CAD build for the part. Positions are in the model's coordinates, mm. Round coordinates to 2 decimals unless told otherwise and drop trailing zeros. Order: outer loops, then holes, each group sorted by start corner. A loop starts at its lowest first (then second) coordinate and runs counter-clockwise, first axis right, second up. Notation, with made-up numbers: (36, 21.25) - (74, 21.25) arc R15 cw to (74, 44.25) - close; hole circle Ø7 at (-23.5, 53). An arc over 180 degrees is marked (long way). Use one line per item in the form item = value. Start each with the question number.
from build123d import *

# Parameters (mm, degrees)
BOSS_EXTRUDE1_DEPTH     = 25
CUT_EXTRUDE1_DEPTH      = 38.279220614
CIRPATTERN1_COUNT       = 8
SHELL2_T                = -10
BOSS_EXTRUDE2_DEPTH     = 15
SKETCH8_R               = 1.75
CUT_EXTRUDE3_DEPTH      = 3.89
SKETCH10_R              = 1.5
CUT_EXTRUDE5_DEPTH      = 10
CIRPATTERN2_COUNT       = 8
CUT_EXTRUDE7_DEPTH      = 2
CUT_EXTRUDE8_DEPTH      = 3.7
FILLET1_R               = 1
CUT_EXTRUDE9_DEPTH      = 1
SKETCH15_R              = 1.1
CUT_EXTRUDE11_DEPTH     = 4
MIRROR2_COPY_1_SKETCH_R = 1.1
MIRROR2_COPY_1_DEPTH    = 4
CUT_EXTRUDE12_DEPTH     = 2.5
SKETCH17_R              = 1
CUT_EXTRUDE13_DEPTH     = 4
CUT_EXTRUDE14_DEPTH     = 0.5
SKETCH19_R              = 3.8
CUT_EXTRUDE15_DEPTH     = 3
CIRPATTERN3_COUNT       = 8


with BuildPart() as part:
    # Sketch3 → Boss-Extrude1 (new body)
    with BuildSketch(Plane(origin=(0, 0, 0), x_dir=(1, 0, 0), z_dir=(0, 1, 0))):
        Polygon((-90, 37.279220614), (-90, -37.279220614), (0, 0), align=None)
    boss_extrude1 = extrude(amount=BOSS_EXTRUDE1_DEPTH)

    # Sketch4 → Cut-Extrude1 (cut, symmetric)
    with BuildSketch(Plane.XY):
        Polygon((-90, 25), (-90, 0), (-80, 25), align=None)
    cut_extrude1 = extrude(amount=CUT_EXTRUDE1_DEPTH, both=True, mode=Mode.SUBTRACT)

    # CirPattern1: Boss-Extrude1, Cut-Extrude1 ×8 about axis
    cirpattern1_axis = Axis((0, 0, 0), (0, 1, 0))
    for i in range(1, CIRPATTERN1_COUNT):
        add(boss_extrude1.rotate(cirpattern1_axis, i * 360 / CIRPATTERN1_COUNT))
        add(cut_extrude1.rotate(cirpattern1_axis, i * 360 / CIRPATTERN1_COUNT), mode=Mode.SUBTRACT)

    # Shell2
    shell2_openings = [part.faces().sort_by_distance(p)[0] for p in [
        (0, 0, 0),
    ]]
    offset(amount=SHELL2_T, openings=shell2_openings, kind=Kind.INTERSECTION)

    # Sketch5 → Boss-Extrude2 (add)
    with BuildSketch(Plane.XZ.offset(-15)):
        with BuildLine():
            Line((-79.229670386, -32.818004016), (-79.229670386, -26.828993349))
            ThreePointArc((-79.229670386, -26.828993349), (-70.654057407, -29.265868815), (-74.99480033, -37.052874072))
            Line((-74.99480033, -37.052874072), (-79.229670386, -32.818004016))
        make_face()
    boss_extrude2 = extrude(amount=BOSS_EXTRUDE2_DEPTH)

    # Sketch8 → Cut-Extrude3 (cut)
    with BuildSketch(Plane.XZ):
        with Locations((-75.906312549, -31.441424128)):
            Circle(SKETCH8_R)
    cut_extrude3 = extrude(amount=-CUT_EXTRUDE3_DEPTH, mode=Mode.SUBTRACT)

    # Sketch10 → Cut-Extrude5 (cut)
    with BuildSketch(Plane.XZ.offset(-3.89)):
        with Locations((-75.906312549, -31.441424128)):
            Circle(SKETCH10_R)
    cut_extrude5 = extrude(amount=-CUT_EXTRUDE5_DEPTH, mode=Mode.SUBTRACT)

    # CirPattern2: Boss-Extrude2, Cut-Extrude3, Cut-Extrude5 ×8 about axis
    cirpattern2_axis = Axis((0, 0, 0), (0, 1, 0))
    for i in range(1, CIRPATTERN2_COUNT):
        add(boss_extrude2.rotate(cirpattern2_axis, i * 360 / CIRPATTERN2_COUNT))
        add(cut_extrude3.rotate(cirpattern2_axis, i * 360 / CIRPATTERN2_COUNT), mode=Mode.SUBTRACT)
        add(cut_extrude5.rotate(cirpattern2_axis, i * 360 / CIRPATTERN2_COUNT), mode=Mode.SUBTRACT)

    # Sketch11 → Cut-Extrude7 (cut)
    with BuildSketch(Plane.XZ.offset(-15)):
        with BuildLine():
            Line((-34.358681844, -65.650070064), (34.041318156, -65.650070064))
            ThreePointArc((34.041318156, -65.650070064), (39.203197659, -63.511949566), (41.341318156, -58.350070064))
            Line((41.341318156, -58.350070064), (41.341318156, -19.050070064))
            ThreePointArc((41.341318156, -19.050070064), (39.203197659, -13.888190561), (34.041318156, -11.750070064))
            Line((34.041318156, -11.750070064), (-34.358681844, -11.750070064))
            ThreePointArc((-34.358681844, -11.750070064), (-39.520561346, -13.888190561), (-41.658681844, -19.050070064))
            Line((-41.658681844, -19.050070064), (-41.658681844, -58.350070064))
            ThreePointArc((-41.658681844, -58.350070064), (-39.520561346, -63.511949566), (-34.358681844, -65.650070064))
        make_face()
        Polygon((26.669250561, 70.01701088), (14.499741046, 57.72095305), (40.157988887, 32.326774235), (52.327498403, 44.622832065), align=None)
        Polygon((-45.807628052, 29.456027416), (-45.557628052, 30.956027416), (-50.265904305, 30.956027416), (-50.015904305, 29.456027416), (-61.961766178, 29.456027416), (-61.961766178, 13.460165542), (-63.461766178, 13.710165542), (-63.461766178, 9.001889289), (-61.961766178, 9.251889289), (-61.961766178, -6.743972584), (20.938233822, -6.743972584), (20.938233822, 10.356027416), (20.938233822, 10.513250754), (20.938233822, 12.198804078), (20.938233822, 12.356027416), (20.938233822, 29.456027416), (8.992371948, 29.456027416), (9.242371948, 30.956027416), (4.534095695, 30.956027416), (4.784095695, 29.456027416), align=None)
        with BuildLine():
            Line((45.394921968, -29.715967357), (66.654814344, -29.648319841))
            ThreePointArc((66.654814344, -29.648319841), (68.279008196, -28.969493954), (68.947484296, -27.341013079))
            Line((68.947484296, -27.341013079), (68.763251409, 30.558693813))
            ThreePointArc((68.763251409, 30.558693813), (68.084425523, 32.182887666), (66.455944648, 32.851363765))
            Line((66.455944648, 32.851363765), (45.196052273, 32.783716249))
            ThreePointArc((45.196052273, 32.783716249), (43.57185842, 32.104890363), (42.903382321, 30.476409488))
            Line((42.903382321, 30.476409488), (43.087615207, -27.423297405))
            ThreePointArc((43.087615207, -27.423297405), (43.766441094, -29.047491257), (45.394921968, -29.715967357))
        make_face()
        Polygon((8.912517718, 34.761532869), (9.383564949, 60.756265326), (-36.708868078, 61.591500425), (-37.179915309, 35.596767968), align=None)
    extrude(amount=-CUT_EXTRUDE7_DEPTH, mode=Mode.SUBTRACT)

    # Sketch13 → Cut-Extrude8 (cut)
    with BuildSketch(Plane.XZ.offset(-17)):
        with BuildLine():
            Line((34.041318156, -11.750070064), (-34.358681844, -11.750070064))
            ThreePointArc((-34.358681844, -11.750070064), (-39.520561346, -13.888190561), (-41.658681844, -19.050070064))
            Line((-41.658681844, -19.050070064), (-41.658681844, -58.350070064))
            ThreePointArc((-41.658681844, -58.350070064), (-39.520561346, -63.511949566), (-34.358681844, -65.650070064))
            Line((-34.358681844, -65.650070064), (34.041318156, -65.650070064))
            ThreePointArc((34.041318156, -65.650070064), (39.203197659, -63.511949566), (41.341318156, -58.350070064))
            Line((41.341318156, -58.350070064), (41.341318156, -19.050070064))
            ThreePointArc((41.341318156, -19.050070064), (39.203197659, -13.888190561), (34.041318156, -11.750070064))
        make_face()
    extrude(amount=-CUT_EXTRUDE8_DEPTH, mode=Mode.SUBTRACT)

    # Fillet1
    fillet1_edges = [part.edges().sort_by_distance(p)[0] for p in [
        (8.912517718, 16, 34.761532869),
        (-37.179915309, 16, 35.596767968),
        (-36.708868078, 16, 61.591500425),
        (9.383564949, 16, 60.756265326),
    ]]
    fillet(fillet1_edges, radius=FILLET1_R)

    # Sketch14 → Cut-Extrude9 (cut)
    with BuildSketch(Plane.XZ.offset(-17)):
        with BuildLine():
            Line((45.394921968, -29.715967357), (66.654814344, -29.648319841))
            ThreePointArc((66.654814344, -29.648319841), (68.279008196, -28.969493954), (68.947484296, -27.341013079))
            Line((68.947484296, -27.341013079), (68.763251409, 30.558693813))
            ThreePointArc((68.763251409, 30.558693813), (68.084425523, 32.182887666), (66.455944648, 32.851363765))
            Line((66.455944648, 32.851363765), (45.196052273, 32.783716249))
            ThreePointArc((45.196052273, 32.783716249), (43.57185842, 32.104890363), (42.903382321, 30.476409488))
            Line((42.903382321, 30.476409488), (43.087615207, -27.423297405))
            ThreePointArc((43.087615207, -27.423297405), (43.766441094, -29.047491257), (45.394921968, -29.715967357))
        make_face()
        Polygon((52.327498403, 44.622832065), (26.669250561, 70.01701088), (14.499741046, 57.72095305), (40.157988887, 32.326774235), align=None)
    extrude(amount=-CUT_EXTRUDE9_DEPTH, mode=Mode.SUBTRACT)

    # Sketch15 → Cut-Extrude11 (cut)
    with BuildSketch(Plane.XZ.offset(-18)):
        with Locations((65.616131079, 29.648675337)):
            Circle(SKETCH15_R)
    cut_extrude11 = extrude(amount=-CUT_EXTRUDE11_DEPTH, mode=Mode.SUBTRACT)

    # Mirror1: Cut-Extrude11 across plane
    add(cut_extrude11.mirror(Plane(origin=(-0.004422036, 0, 1.38973325), x_dir=(0.999994938, 0, 0.003181915), z_dir=(0.003181915, 0, -0.999994938))), mode=Mode.SUBTRACT)

    # Mirror2: Cut-Extrude11 across plane
    add(cut_extrude11.mirror(Plane(origin=(55.929855344, 0, 0.177964954), x_dir=(-0.003181915, 0, 0.999994938), z_dir=(-0.999994938, 0, -0.003181915))), mode=Mode.SUBTRACT)

    # Mirror2 copy 1 sketch → Mirror2 copy 1 (cut)
    with BuildSketch(Plane(origin=(111.850866616, 18, 3.135396408), x_dir=(-1, 0, 0), z_dir=(0, -1, 0))):
        with Locations((65.616131079, 29.648675337)):
            Circle(MIRROR2_COPY_1_SKETCH_R)
    extrude(amount=-MIRROR2_COPY_1_DEPTH, mode=Mode.SUBTRACT)

    # Sketch16 → Cut-Extrude12 (cut)
    with BuildSketch(Plane.XZ.offset(-17)):
        Polygon((4.784095695, 29.456027416), (-45.807628052, 29.456027416), (-45.557628052, 30.956027416), (-50.265904305, 30.956027416), (-50.015904305, 29.456027416), (-61.961766178, 29.456027416), (-61.961766178, 13.460165542), (-63.461766178, 13.710165542), (-63.461766178, 9.001889289), (-61.961766178, 9.251889289), (-61.961766178, -6.743972584), (20.938233822, -6.743972584), (20.938233822, 29.456027416), (8.992371948, 29.456027416), (9.242371948, 30.956027416), (4.534095695, 30.956027416), align=None)
    extrude(amount=-CUT_EXTRUDE12_DEPTH, mode=Mode.SUBTRACT)

    # Sketch17 → Cut-Extrude13 (cut)
    with BuildSketch(Plane.XZ.offset(-18)):
        with Locations((18.389142064, 57.67035938)):
            Circle(SKETCH17_R)
        with Locations((40.067163093, 36.21544376)):
            Circle(SKETCH17_R)
    extrude(amount=-CUT_EXTRUDE13_DEPTH, mode=Mode.SUBTRACT)

    # Sketch18 → Cut-Extrude14 (cut)
    with BuildSketch(Plane.XZ.offset(-17)):
        with BuildLine():
            Line((8.930635616, 35.761368726), (9.365447051, 59.756429468))
            ThreePointArc((9.365447051, 59.756429468), (9.085413197, 60.468726793), (8.383729092, 60.774383224))
            Line((8.383729092, 60.774383224), (-35.70903222, 61.573382527))
            ThreePointArc((-35.70903222, 61.573382527), (-36.421329544, 61.293348673), (-36.726985976, 60.591664568))
            Line((-36.726985976, 60.591664568), (-37.16179741, 36.596603826))
            ThreePointArc((-37.16179741, 36.596603826), (-36.881763556, 35.884306501), (-36.180079451, 35.57865007))
            Line((-36.180079451, 35.57865007), (7.912681861, 34.779650767))
            ThreePointArc((7.912681861, 34.779650767), (8.624979185, 35.059684621), (8.930635616, 35.761368726))
        make_face()
    extrude(amount=-CUT_EXTRUDE14_DEPTH, mode=Mode.SUBTRACT)

    # Sketch19 → Cut-Extrude15 (cut)
    with BuildSketch(Plane.XZ):
        with Locations((52.760655942, -66.902791566)):
            Circle(SKETCH19_R)
        with Locations((66.902791566, -52.760655942)):
            Circle(SKETCH19_R)
    cut_extrude15 = extrude(amount=-CUT_EXTRUDE15_DEPTH, mode=Mode.SUBTRACT)

    # CirPattern3: Cut-Extrude15 ×8 about axis, 2 skipped
    cirpattern3_axis = Axis((0, 0, 0), (0, 1, 0))
    add([cut_extrude15.rotate(cirpattern3_axis, i * 360 / CIRPATTERN3_COUNT) for i in range(1, CIRPATTERN3_COUNT) if i not in (3, 7)], mode=Mode.SUBTRACT)


solid = part.part
(1) Mould opens along X. For faces 1 (the flat face through (-0.52, 12.32, -85.07)), 2 (the cylindrical face through (56.385, 1.479, -65.761)), 3 (the flat face through (85.07, 12.32, -0.52)), 4 (the flat face through (-59.785, 12.325, 60.523)) say: pulls with the +X half, pulls with the -X half, needs draft (parallel to the pull), parting line crosses it, or undercut.
(2) Flat gauge pins, fed straight in: P1, Ø1, axis at y = 20.5, z = -13, coming from the -X side; P2, Ø1, axis at x = -55.5, y = 7.5, coming from the +Z side; P3, Ø8, axis at x = -2.5, z = 14, coming from the -Y side. Where does each tip first touch, or does it go through?
(3) Slice it at C-C (x = -10). Give the cut face in (y, z).
(4) Slice it at B-B (z = -1). Give the cut face in (x, y), and give its area (3 significant figures).
(5) Wall check: line 1 (Z direction, x = -51.5, y = 2.25); line 2 (X direction, y = 3.5, z = 77); line 3 (X direction, y = 15.75, z = -16). Give the ranges that are in metal, low to high. Write a range as [from, to].
(6) Slice it at A-A (y = 7.5). Give the number of separate pieces and of enclosed holes in the cut face, and give its area (3 significant figures).
Results list:
q1.face_1 = needs draft
q1.face_2 = undercut
q1.face_3 = pulls with the +X half
q1.face_4 = pulls with the -X half
q2.P1 = -82
q2.P2 = 68.11
q2.P3 = 19.5
q3.outline = (0, -90) - (25, -80) - (25, 80) - (0, 90) - (0, 88.41) - (3, 88.41) - (3, 80.81) - (0, 80.81) - (0, 79.23) - (15, 73.23) - (15, 61.11) - (17.5, 61.11) - (17.5, 35.1) - (15, 35.1) - (15, 29.46) - (19.5, 29.46) - (19.5, -6.74) - (15, -6.74) - (15, -11.75) - (20.7, -11.75) - (20.7, -65.65) - (15, -65.65) - (15, -73.23) - (0, -79.23) - (0, -80.81) - (3, -80.81) - (3, -88.41) - (0, -88.41) - close
q4.outline = (-90, 0) - (-79.23, 0) - (-73.23, 15) - (-61.96, 15) - (-61.96, 19.5) - (20.94, 19.5) - (20.94, 15) - (43, 15) - (43, 18) - (68.86, 18) - (68.86, 15) - (73.23, 15) - (79.23, 0) - (90, 0) - (80, 25) - (-80, 25) - close
q4.area = 1,510 mm²
q5.line_1 = [-74.51, -70.49], [-63.32, -59.27], [59.27, 63.32], [70.49, 74.51]
q5.line_2 = [-48.3, -32.81], [-30.08, -25.86], [25.86, 30.08], [32.81, 48.3]
q5.line_3 = [-83.7, -40.99], [40.67, 43.05], [68.91, 83.7]
q6.separate_pieces = 1
q6.enclosed_holes = 9
q6.area = 6,100 mm²
